Verification items for this drawing (mm, ordinates from the low corner). A direction names the side the tool comes from. Round coordinates to 2 decimals unless told otherwise and drop trailing zeros. Loops run counter-clockwise (first coordinate to the right, second up) from the corner with the lowest first, then second, coordinate; pieces in that order, holes last. Notation, with made-up numbers: M -35.5,-23.5 L -14.5,-23.5 A18 cw -14.5,-3.5 Z; hole C 58,-26 d6. An arc over 180 degrees is marked long. Write item = value, one per line. Start each with the question number.
(1) Cross-section at A-A on y = 10. Record the boundary of the cut face in (x, z), plus the area to 3 significant figures.
(2) Go/stop test with flat-tipped pins: P1, Ø10, axis at x = 17, y = 3.5, coming from the +Z side; P2, Ø12, axis at x = 3.5, z = 11.5, coming from the -Y side; P3, Ø4, axis at x = 10.5, y = 10.5, coming from the -Z side. Record where each tip stops, or that it passes through.
(3) Scan lines: L1, parallel to Y at x = 10, z = 5.55; L2, parallel to Z at x = 11.75, y = 8; L3, parallel to Y at x = 10.25, z = 16.75. Record each from-to range of solid material in increasing order. Write a range as from..to.
(4) Set-up check for the marked faces 1, 2 and 3: record each of +Z, -Z, +X, -X, +Y, -Y from which the full face is reachable in a straight line by a thin tool's end or side.
(5) Cross-section at D-D on y = 5.5. Record the boundary of the cut face in (x, z).
(6) Cross-section at C-C on z = 14.25. Record the boundary of the cut face in (x, y).
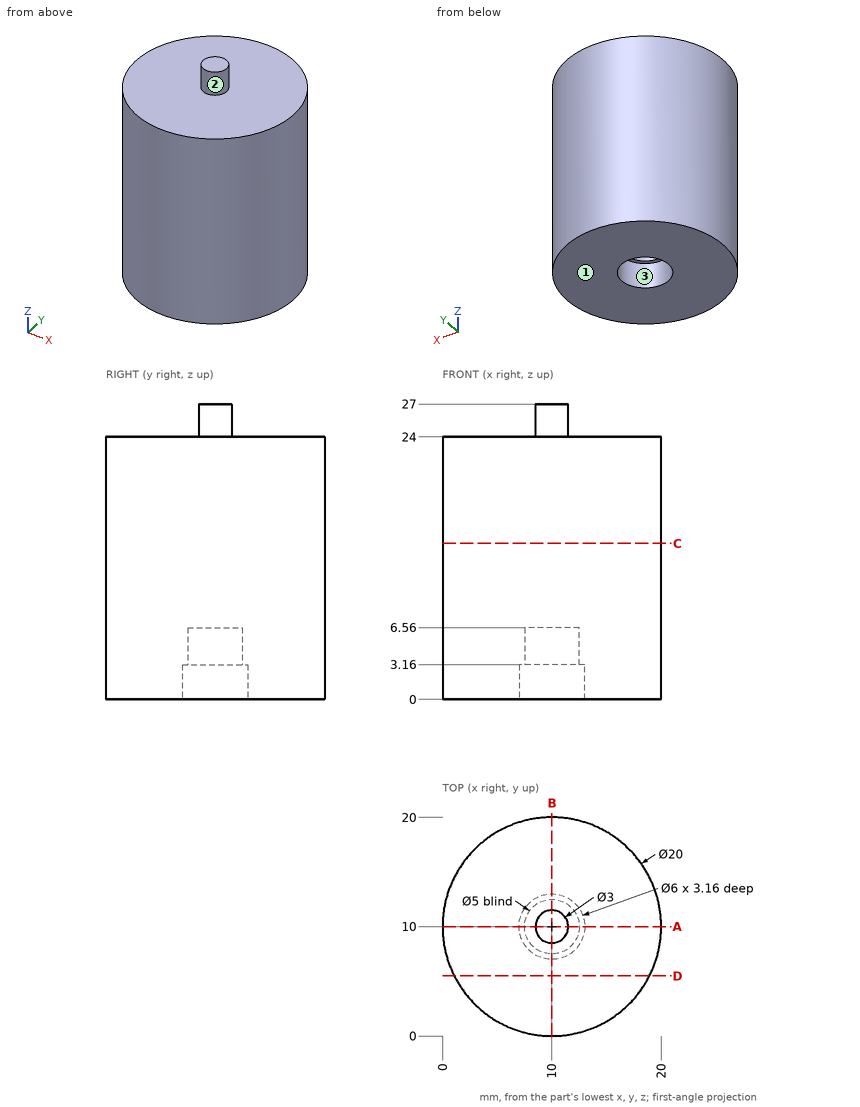
Result:
q1.outline = M 0,0 L 7,0 L 7,3.16 L 7.5,3.16 L 7.5,6.56 L 12.5,6.56 L 12.5,3.16 L 13,3.16 L 13,0 L 20,0 L 20,24 L 11.5,24 L 11.5,27 L 8.5,27 L 8.5,24 L 0,24 Z
q1.area = 453 mm^2
q2.P1 = 24
q2.P2 = 0.01
q2.P3 = 3.16
q3.L1 = 0..7.5, 12.5..20
q3.L2 = 3.16..24
q3.L3 = 0..20
q4.face_1 = -Z, +X, -X, +Y, -Y
q4.face_2 = +Z
q4.face_3 = -Z
q5.outline = M 1.07,0 L 18.93,0 L 18.93,24 L 1.07,24 Z
q6.outline = C 10,10 d20
